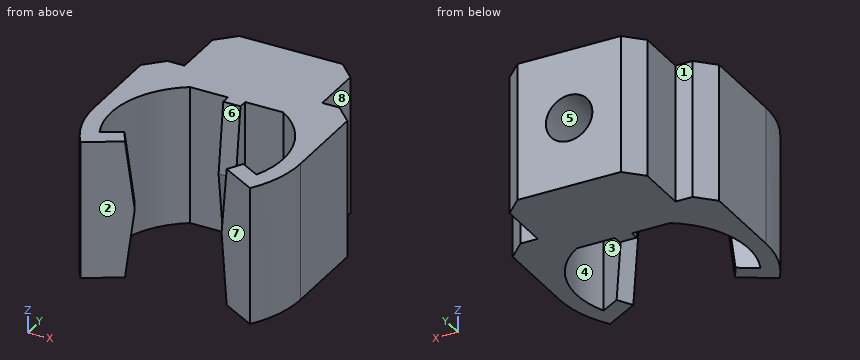
```python
from build123d import *
from OCP.BRepFilletAPI import BRepFilletAPI_MakeChamfer

# Parameters (mm, degrees)
BOSS_EXTRUDE2_DEPTH = 8
SKETCH11_R          = 1.35
CUT_EXTRUDE5_DEPTH  = 5
CHAMFER1_SIZE       = 1
CHAMFER2_SIZE       = 4
CHAMFER2_SIZE_2     = 0.5
CHAMFER3_SIZE       = 0.5
CHAMFER3_SIZE2      = 4


with BuildPart() as part:
    # Sketch1 → Boss-Extrude2 (new body)
    with BuildSketch(Plane.XY):
        with BuildLine():
            Line((-2.712931993, 4.2), (-0.5, 4.2))
            Line((-0.5, 4.2), (-0.5, 3.2))
            Line((-0.5, 3.2), (0.5, 3.2))
            Line((0.5, 3.2), (0.5, 4.2))
            Line((0.5, 4.2), (2.712931993, 4.2))
            ThreePointArc((2.712931993, 4.2), (4.795591913, 1.415025868), (4.558421985, -2.054455891))
            Line((4.558421985, -2.054455891), (3.021281292, -1.166987298))
            Line((3.021281292, -1.166987298), (2.521281292, -2.033012702))
            Line((2.521281292, -2.033012702), (4.928078794, -3.422577888))
            ThreePointArc((4.928078794, -3.422577888), (5.725752036, -1.793255034), (6, 0))
            Line((6, 0), (6, 6))
            Line((6, 6), (4, 6))
            Line((4, 6), (4, 10))
            Line((4, 10), (-4, 10))
            Line((-4, 10), (-4, 6))
            Line((-4, 6), (-6, 6))
            Line((-6, 6), (-6, 0))
            ThreePointArc((-6, 0), (-5.725752036, -1.793255034), (-4.928078794, -3.422577888))
            Line((-4.928078794, -3.422577888), (-2.521281292, -2.033012702))
            Line((-2.521281292, -2.033012702), (-3.021281292, -1.166987298))
            Line((-3.021281292, -1.166987298), (-4.558421985, -2.054455891))
            ThreePointArc((-4.558421985, -2.054455891), (-4.795591913, 1.415025868), (-2.712931993, 4.2))
        make_face()
    extrude(amount=BOSS_EXTRUDE2_DEPTH)

    # Sketch11 → Cut-Extrude5 (cut)
    with BuildSketch(Plane(origin=(0, 10, 0), x_dir=(1, 0, 0), z_dir=(0, 1, 0))):
        with Locations(Location((0, -4, 0), (0, 0, 270))):
            Circle(SKETCH11_R)
    extrude(amount=-CUT_EXTRUDE5_DEPTH, mode=Mode.SUBTRACT)

    # Chamfer1
    chamfer1_edges = [part.edges().sort_by_distance(p)[0] for p in [
        (-6, 6, 4),
        (-4, 10, 4),
        (4, 10, 4),
        (6, 6, 4),
    ]]
    chamfer(chamfer1_edges, length=CHAMFER1_SIZE)

    # Chamfer2
    chamfer2_edges_1 = [part.edges().sort_by_distance(p)[0] for p in [
        (2.771281292, -1.6, 8),
    ]]
    chamfer2_side_1 = [part.faces().sort_by_distance(p)[0] for p in [
        (2.771281292, -1.6, 7.99),
    ]]
    chamfer2_edges_2 = [part.edges().sort_by_distance(p)[0] for p in [
        (2.771281292, -1.6, 0),
    ]]
    chamfer2_side_2 = [part.faces().sort_by_distance(p)[0] for p in [
        (2.779941546, -1.605, 0),
    ]]
    chamfer2_edges_3 = [part.edges().sort_by_distance(p)[0] for p in [
        (0, 3.2, 8),
    ]]
    chamfer2_side_3 = [part.faces().sort_by_distance(p)[0] for p in [
        (0, 3.2, 7.99),
    ]]
    chamfer2_edges_4 = [part.edges().sort_by_distance(p)[0] for p in [
        (-2.771281292, -1.6, 8),
    ]]
    chamfer2_side_4 = [part.faces().sort_by_distance(p)[0] for p in [
        (-2.771281292, -1.6, 7.99),
    ]]
    chamfer2 = BRepFilletAPI_MakeChamfer(part.part.solid().wrapped)
    for e in chamfer2_edges_1:
        chamfer2.Add(CHAMFER2_SIZE - 0.0001, CHAMFER2_SIZE_2 - 0.0001, e.wrapped, chamfer2_side_1[0].wrapped)
    for e in chamfer2_edges_2:
        chamfer2.Add(CHAMFER2_SIZE_2 - 0.0001, CHAMFER2_SIZE - 0.0001, e.wrapped, chamfer2_side_2[0].wrapped)
    for e in chamfer2_edges_3:
        chamfer2.Add(CHAMFER2_SIZE - 0.0001, CHAMFER2_SIZE_2 - 0.0001, e.wrapped, chamfer2_side_3[0].wrapped)
    for e in chamfer2_edges_4:
        chamfer2.Add(CHAMFER2_SIZE - 0.0001, CHAMFER2_SIZE_2 - 0.0001, e.wrapped, chamfer2_side_4[0].wrapped)
    add(Compound.cast(chamfer2.Shape()), mode=Mode.REPLACE)  # a hair under: the kernel refuses the full size

    # Chamfer3
    chamfer3_edges = [part.edges().sort_by_distance(p)[0] for p in [
        (-2.771281292, -1.6, 0),
        (0, 3.2, 0),
    ]]
    chamfer3_side = [part.faces().sort_by_distance(p)[0] for p in [
        (-0.019519244, 4.871717055, 0),
    ]]
    chamfer(chamfer3_edges, length=CHAMFER3_SIZE, length2=CHAMFER3_SIZE2, reference=chamfer3_side[0])


solid = part.part
```
The model under review builds one solid part; all positions refer to its coordinate system, in mm. Face numbers are marked on the shaded views. A direction names the side the tool comes from. Give positions to 0.01 mm unless a question says otherwise; leave off trailing zeros. Loops run counter-clockwise (first coordinate to the right, second up) from the corner with the lowest first, then second, coordinate; pieces in that order, holes last. Notation, with made-up numbers: (79.25, 50) - (114.25, 50) arc R29 cw to (114.25, 89) - close; hole circle Ø6 at (4.25, -35.5). An arc over 180 degrees is marked (long way). Answer as a JSON object with one key per item and string values.
Q1. Add section C-C on x = -3.25. State the section outline as (y, z) points, plus the area to 4 significant figures.
Worked out:
{"outline": "(-2.45, 0) - (-1.77, 0) - (-1.3, 1.89) - (-1.3, 6.11) - (-1.77, 8) - (-2.45, 8) - close; (3.8, 0) - (9.75, 0) - (9.75, 8) - (3.8, 8) - close", "area": "55.95 mm^2"}
Q2. Add section D-D on z = 1.25. State the section outline as (x, y) points.
Worked out:
{"outline": "(-6, 0) arc R6 ccw to (-4.93, -3.42) - (-2.82, -2.2) - (-3.32, -1.34) - (-4.56, -2.05) arc R5 cw to (-2.71, 4.2) - (-0.5, 4.2) - (-0.5, 3.54) - (0.5, 3.54) - (0.5, 4.2) - (2.71, 4.2) arc R5 cw to (4.56, -2.05) - (3.32, -1.34) - (2.82, -2.2) - (4.93, -3.42) arc R6 ccw to (6, 0) - (6, 5) - (5, 6) - (4, 6) - (4, 9) - (3, 10) - (-3, 10) - (-4, 9) - (-4, 6) - (-5, 6) - (-6, 5) - close"}
Q3. To check wall thickness, follow line 1 along X through (y, z) = (7.5, 4); line 2 along X through (y, z) = (3, 3); line 3 along X through (y, z) = (6.5, 1). State the ranges of each line that lie inside material, in increasing order.
Worked out:
{"line 1": "x = -4 to -1.35, 1.35 to 4", "line 2": "x = -6 to -4, 4 to 6", "line 3": "x = -4 to 4"}
Q4. Add section A-A on y = 2.75. State the section outline as (x, z) points.
Worked out:
{"outline": "(-6, 0) - (-4.18, 0) - (-4.18, 8) - (-6, 8) - close; (4.18, 0) - (6, 0) - (6, 8) - (4.18, 8) - close"}
Q5. For the marked faces 4, 5, 6, 7 and 8, list the 3-axis set-ups (+Z, -Z, +X, -X, +Y, -Y) from which the entire face can be reached by the end or side of a thin tool; tool diameter is ignored.
Worked out:
{"face 4": "+Z, -Z", "face 5": "+Y", "face 6": "+Z, -Y", "face 7": "+Z, -Z, -Y", "face 8": "+Z, -Z, +X, +Y"}
Q6. Add section B-B on y = 8. State the section outline as (x, z) points, plus the area to 3 significant figures.
Worked out:
{"outline": "(-4, 0) - (4, 0) - (4, 8) - (-4, 8) - close; hole circle Ø2.7 at (0, 4)", "area": "58.3 mm^2"}
Q7. Insertion check: pin 1 (0.8 mm diameter, centred on x = 4.5, z = 2, fed in from +Y); pin 2 (3.5 mm diameter, centred on y = 7, z = 3.5, fed in from -X); pin 3 (1.8 mm diameter, centred on x = 1, z = 2, fed in from -Y). Each pin has a flat end and moves straight along its axis. Give the tip position at first contact, or say it passes through.
Worked out:
{"pin 1": "stops at y = 6", "pin 2": "stops at x = -5.75", "pin 3": "stops at y = 3.36"}
Q8. Mouldability with a two-part tool opening along Y and no side actions: class the marked faces 1, 2 and 3 as +Y half, -Y half, draft (parallel to the pull), parting line (faces both ways), or undercut.
Worked out:
{"face 1": "+Y half", "face 2": "-Y half", "face 3": "undercut"}
